Job drawing, mm, ordinate dimensions from the low corner. One solid piece. Round coordinates to 2 decimals unless told otherwise and drop trailing zeros. Order: outer loops, then holes, each group sorted by start corner. A loop starts at its lowest first (then second) coordinate and runs counter-clockwise, first axis right, second up. Notation, with made-up numbers: (59.25, -31) - (102.25, -31) arc R15 cw to (102.25, -20) - close; hole circle Ø2 at (10.25, 16). An arc over 180 degrees is marked (long way). Write each question's results on one line, items separated by ' | '. Start each with the question number.
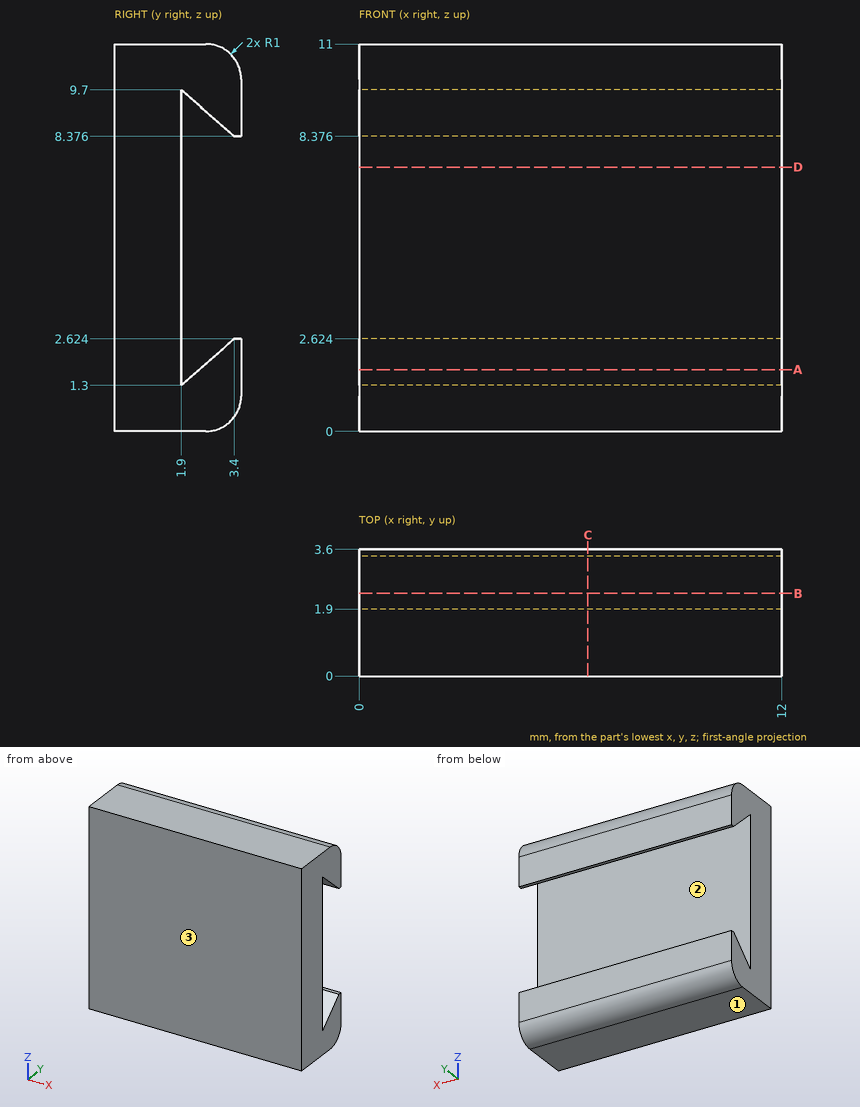
1. Flat gauge pin, fed straight in: pin 1 Ø5 at (x, z) = (3, 3) entering from -Y. Where does the tip first touch, or does it go through?
2. Cut at C-C (x = 6.5). List the corners of the cut face in (y, z), plus the area to 3 significant figures.
3. Wall check: line 1 (Y direction, x = 0.5, z = 6.5); line 2 (Y direction, x = 3.25, z = 8.5); line 3 (Y direction, x = 5.25, z = 1.5) (1 decimal). Give the ranges that are in metal, low to high. Write a range as from..to.
4. Cut at B-B (y = 2.35). List the corners of the cut face in (x, z).
5. Cut at D-D (z = 7.5). List the corners of the cut face in (x, y).
6. Cut at A-A (z = 1.75). List the corners of the cut face in (x, y).
7. Mould opens along Z. For the marked faces 1, 2 and 3 say: pulls with the +Z half, pulls with the -Z half, needs draft (parallel to the pull), parting line crosses it, or undercut.
A:
1) pin 1: stops at y = 0
2) outline: (0, 0) - (2.6, 0) arc R1 ccw to (3.6, 1) - (3.6, 2.62) - (3.4, 2.62) - (1.9, 1.3) - (1.9, 9.7) - (3.4, 8.38) - (3.6, 8.38) - (3.6, 10) arc R1 ccw to (2.6, 11) - (0, 11) - close | area: 27.4 mm^2
3) line 1: y = 0..1.9 | line 2: y = 0..1.9, 3.26..3.6 | line 3: y = 0..1.9, 2.1..3.6
4) outline: (0, 0) - (12, 0) - (12, 1.7) - (0, 1.7) - close; (0, 9.3) - (12, 9.3) - (12, 11) - (0, 11) - close
5) outline: (0, 0) - (12, 0) - (12, 1.9) - (0, 1.9) - close
6) outline: (0, 0) - (12, 0) - (12, 1.9) - (0, 1.9) - close; (0, 2.41) - (12, 2.41) - (12, 3.6) - (0, 3.6) - close
7) face 1: pulls with the -Z half | face 2: undercut | face 3: needs draft
